Geometry: final body of the model. Coordinates: model frame, mm. A direction names the side the tool comes from. Give positions to 0.01 mm unless a question says otherwise; leave off trailing zeros. Loops run counter-clockwise (first coordinate to the right, second up) from the corner with the lowest first, then second, coordinate; pieces in that order, holes last. Notation, with made-up numbers: (54.5, 29) -> (105.5, 29) arc R35 ccw to (105.5, 62) -> close; hole circle Ø7 at (-19, -20). An arc over 180 degrees is marked (long way). Answer in a Markdown table with one row per item. Add a question column.
1) Draft query along Y for faces 4 (the flat face through (5.504, 6, 17)), 5 (the flat face through (-1, 0, -6)), 6 (the cylindrical face through (2.45, 7.23, -17.65)), 7 (the cylindrical face through (-11.026, 6.951, 16.995)). Return one class per face: +Y half, -Y half, draft (parallel to the pull), parting line (faces both ways), or undercut.
2) Section query A-A (y = 6.35). Return the cut outline in (x, z) (1 decimal), plus the area to 3 significant figures.
3) First-contact query: P1, Ø6.5, axis at y = 4.5, z = -20.5, coming from the +X side; P2, Ø1.1, axis at x = 2.33, y = 6.35, coming from the +Z side; P3, Ø2, axis at x = -1, z = -9.5, coming from the +Y side; P4, Ø11.5, axis at x = -4.02, z = 0, coming from the -Y side. Flat tips, straight axial feed; report the tip coordinate or a pass-through.
4) Access query for faces 1 (the flat face through (5.504, 6, -17)), 2 (the cylindrical face through (2.21, 7.23, 17)), 3 (the flat face through (-10, 6, -10.649)). Directions: +Z, -Z, +X, -X, +Y, -Y. A direction counts if a zero-diameter tool reaches every point of the face in a straight line with its end or side. Return the directions, or none.
5) Section query D-D (y = 9.5). Return the cut outline in (x, z) (1 decimal), plus the area to 3 significant figures.
6) Section query C-C (z = -14). Return the cut outline in (x, y), plus the area to 3 significant figures.
7) Line query: line 1 (X direction, y = 6, z = -18.5); line 2 (X direction, y = 3, z = -11.5); line 3 (Y direction, x = 2.5, z = -20.5). Output: solid intervals per line, ascending. Write a range as from..to.
8) Section query B-B (z = 0). Return the cut outline in (x, y).
Autodesk Inventor part; units mm, degrees
ref_plane "YZ Plane" through (0, 0, 0) normal (1, 0, 0) x (0, 1, 0)
ref_plane "XZ Plane" through (0, 0, 0) normal (0, 1, 0) x (-1, 0, 0)
ref_plane "XY Plane" through (0, 0, 0) normal (0, 0, 1) x (1, 0, 0)
sketch "Sketch1" plane through (0, 0, 0) normal (0, 1, 0) x (-1, 0, 0)
  line L0 (13.5456, 23.1663) -> (-5.5044, 23.1663)
  line L1 (-5.5044, -24.4587) -> (13.5456, -24.4587)
  line L2 (-5.5044, 23.1663) -> (-5.5044, 10.6493)
  line L3 (-5.5044, -10.6493) -> (-5.5044, -24.4587)
  line L4 (13.5456, -24.4587) -> (13.5456, -10.6493)
  line L5 (13.5456, 10.6493) -> (13.5456, 23.1663)
  circle A0 centre (4.0206, 0) radius 6.35
  arc A1 (13.5456, -10.6493) -> (13.5456, 10.6493) centre (4.0206, 0) ccw
  arc A2 (-5.5044, 10.6493) -> (-5.5044, -10.6493) centre (4.0206, 0) ccw
  point P0 (0, 0)
  dimension "d0" = 47.625
  dimension "d1" = 19.05
  dimension "d3" = 12.7
extrude "Extrusion1" add sketch "Sketch1" along normal blind 12.7
sketch "Sketch2" plane through (0, 12.7, 0) normal (0, 1, 0) x (1, 0, 0)
  circle A0 centre (-4.0206, 0) radius 6.35
  circle A1 centre (-4.0206, 0) radius 11.1125
  point P0 (0, 0)
  dimension "d7" = 22.225
extrude "Extrusion2" cut sketch "Sketch2" against normal blind 7.112
sketch "Sketch3" plane through (-13.5456, 0, 23.1663) normal (0, 0, 1) x (1, 0, 0)
  line L0 (0, 0) -> (0, 12.7)
  line L1 (19.05, 0) -> (19.05, 12.7)
  circle A0 centre (3.175, 6.35) radius 0.889
  circle A1 centre (15.875, 6.35) radius 0.889
  point P0 (13.5456, 0)
  dimension "d10" = 3.175
  dimension "d11" = 3.175
  dimension "d12" = 1.778
  dimension "d13" = 1.778
extrude "Extrusion3" cut sketch "Sketch3" against normal up to surface (12.5171 mm away)
sketch "Sketch4" plane through (5.5044, 0, -24.4587) normal (0, 0, -1) x (-1, 0, 0)
  circle A0 centre (3.175, 6.35) radius 0.889
  circle A1 centre (15.875, 6.35) radius 0.889
  point P0 (5.5044, 0)
extrude "Extrusion4" cut sketch "Sketch4" against normal up to surface (13.8094 mm away)
properties part number "top_anchor"
Evaluation:
| question | item | result |
|---|---|---|
| 1 | face 4 | draft |
| 1 | face 5 | -Y half |
| 1 | face 6 | undercut |
| 1 | face 7 | undercut |
| 2 | outline | (-13.5, -24.5) -> (-11.3, -24.5) -> (-11.3, -10.6) -> (-9.5, -10.6) -> (-9.5, -24.5) -> (1.4, -24.5) -> (1.4, -10.6) -> (3.2, -10.6) -> (3.2, -24.5) -> (5.5, -24.5) -> (5.5, -10.6) arc R14.3 ccw to (5.5, 10.6) -> (5.5, 23.2) -> (3.2, 23.2) -> (3.2, 10.6) -> (1.4, 10.6) -> (1.4, 23.2) -> (-9.5, 23.2) -> (-9.5, 10.6) -> (-11.3, 10.6) -> (-11.3, 23.2) -> (-13.5, 23.2) -> (-13.5, 10.6) arc R14.3 ccw to (-13.5, -10.6) -> close; hole circle Ø22.2 at (-4, 0) |
| 2 | area | 566 mm² |
| 3 | P1 | x = 5.5 |
| 3 | P2 | z = 10.65 |
| 3 | P3 | y = 5.59 |
| 3 | P4 | through |
| 4 | face 1 | -Z, +X, +Y, -Y |
| 4 | face 2 | +Z |
| 4 | face 3 | -Z |
| 5 | outline | (-13.5, -24.5) -> (5.5, -24.5) -> (5.5, -10.6) arc R14.3 ccw to (5.5, 10.6) -> (5.5, 23.2) -> (-13.5, 23.2) -> (-13.5, 10.6) arc R14.3 ccw to (-13.5, -10.6) -> close; hole circle Ø22.2 at (-4, 0) |
| 5 | area | 660 mm² |
| 6 | outline | (-13.55, 0) -> (5.5, 0) -> (5.5, 12.7) -> (-13.55, 12.7) -> close; hole circle Ø1.78 at (-10.37, 6.35); hole circle Ø1.78 at (2.33, 6.35) |
| 6 | area | 237 mm² |
| 7 | line 1 | -13.55..-11.19, -9.55..1.51, 3.15..5.5 |
| 7 | line 2 | -13.55..5.5 |
| 7 | line 3 | 0..5.48, 7.22..12.7 |
| 8 | outline | (-18.31, 0) -> (-10.37, 0) -> (-10.37, 5.59) -> (-15.13, 5.59) -> (-15.13, 12.7) -> (-18.31, 12.7) -> close; (2.33, 0) -> (10.27, 0) -> (10.27, 12.7) -> (7.09, 12.7) -> (7.09, 5.59) -> (2.33, 5.59) -> close |
